from build123d import *

# Parameters (mm, degrees)
SKETCH1_R                  = 35
SKETCH1_R_2                = 13
SKETCH1_R_3                = 5
SKETCH1_R_4                = 2.3
SKETCH1_W                  = 47.96
SKETCH1_H                  = 25
BOSS_EXTRUDE3_DEPTH        = 5.588
F_4_6_4_6_DIAMETER_HOLE1_D = 4.6
FILLET1_R                  = 3
FILLET2_R                  = 2
FILLET3_R                  = 2
FILLET4_R                  = 1
SKETCH6_W                  = 55.082421743
SKETCH6_H                  = 3.3
CUT_EXTRUDE5_DEPTH         = 10
SKETCH7_W                  = 1.65
SKETCH7_H                  = 1.65
BOSS_EXTRUDE4_DEPTH        = 5.588
FILLET5_R                  = 1
FILLET6_R                  = 0.5
FILLET7_R                  = 0.5
FILLET11_R                 = 1
FILLET13_R                 = 0.1
FILLET14_R                 = 0.1


with BuildPart() as part:
    # Sketch1 → Boss-Extrude3 (new body)
    # profile 1 of 5: a face of its own
    with BuildSketch(Plane(origin=(0, 0, 0), x_dir=(1, 0, 0), z_dir=(0, 1, 0))):
        with Locations((32.785, 23.351471482)):
            Circle(SKETCH1_R)
        with Locations(Location((32.785, 23.351471482, 0), (0, 0, 270))):
            Circle(SKETCH1_R_2, mode=Mode.SUBTRACT)
    # profile 2 of 5: a face of its own
    with BuildSketch(Plane(origin=(0, 0, 0), x_dir=(1, 0, 0), z_dir=(0, 1, 0))):
        with Locations((65.600049901, 5.201471482)):
            Circle(SKETCH1_R_3)
        with Locations(Location((65.600049901, 5.201471482, 0), (0, 0, 270))):
            Circle(SKETCH1_R_4, mode=Mode.SUBTRACT)
    # profile 3 of 5: a face of its own
    with BuildSketch(Plane(origin=(0, 0, 0), x_dir=(1, 0, 0), z_dir=(0, 1, 0))):
        with Locations((-0.030049901, 5.201471482)):
            Circle(SKETCH1_R_3)
        with Locations(Location((-0.030049901, 5.201471482, 0), (0, 0, 270))):
            Circle(SKETCH1_R_4, mode=Mode.SUBTRACT)
    # profile 4 of 5: a face of its own
    with BuildSketch(Plane(origin=(0, 0, 0), x_dir=(1, 0, 0), z_dir=(0, 1, 0))):
        with Locations((32.785, 68.701471482)):
            Circle(SKETCH1_R_3)
    # profile 5 of 5: a face of its own
    with BuildSketch(Plane(origin=(0, 0, 0), x_dir=(1, 0, 0), z_dir=(0, 1, 0))):
        with Locations((32.785, 54.201471482)):
            Rectangle(SKETCH1_W, SKETCH1_H)
    extrude(amount=BOSS_EXTRUDE3_DEPTH)

    # Ø4.6 (4.6) Diameter Hole1 (through all)
    with Locations(Plane(origin=(0, 5.588, 0), x_dir=(1, 0, 0), z_dir=(0, 1, 0))):
        with Locations((32.785, 68.701471482)):
            Hole(F_4_6_4_6_DIAMETER_HOLE1_D / 2)

    # Fillet1
    fillet1_edges = [part.edges().sort_by_distance(p)[0] for p in [
        (65.214711372, 2.794, -10.18660079),
        (61.172514444, 2.794, -2.878342174),
        (0.355288628, 2.794, -10.18660079),
        (4.397485556, 2.794, -2.878342174),
    ]]
    fillet(fillet1_edges, radius=FILLET1_R)

    # Fillet2
    fillet2_edges = [part.edges().sort_by_distance(p)[0] for p in [
        (28.202424305, 2.794, -66.701471482),
        (37.367575695, 2.794, -66.701471482),
    ]]
    fillet(fillet2_edges, radius=FILLET2_R)

    # Fillet3
    fillet3_edges = [part.edges().sort_by_distance(p)[0] for p in [
        (8.805, 2.794, -48.845776728),
        (56.765, 2.794, -48.845776728),
    ]]
    fillet(fillet3_edges, radius=FILLET3_R)

    # Fillet4
    fillet4_edges = [part.edges().sort_by_distance(p)[0] for p in [
        (56.765, 2.794, -66.701471482),
        (8.805, 2.794, -66.701471482),
    ]]
    fillet(fillet4_edges, radius=FILLET4_R)

    # Sketch6 → Cut-Extrude5 (cut)
    with BuildSketch(Plane(origin=(0, 5.588, 0), x_dir=(1, 0, 0), z_dir=(0, 1, 0))):
        with Locations((41.000226715, 37.751471482)):
            Rectangle(SKETCH6_W, SKETCH6_H)
    extrude(amount=-CUT_EXTRUDE5_DEPTH, mode=Mode.SUBTRACT)

    # Sketch7 → Boss-Extrude4 (add)
    with BuildSketch(Plane(origin=(0, 5.588, 0), x_dir=(1, 0, 0), z_dir=(0, 1, 0))):
        with Locations((40.61, 38.576471482)):
            Rectangle(SKETCH7_W, SKETCH7_H)
        with Locations((25.56, 38.576471482)):
            Rectangle(SKETCH7_W, SKETCH7_H)
    extrude(amount=-BOSS_EXTRUDE4_DEPTH)

    # Fillet5
    fillet5_edges = [part.edges().sort_by_distance(p)[0] for p in [
        (13.459015843, 2.794, -36.101471482),
        (13.459015843, 2.794, -39.401471482),
    ]]
    fillet(fillet5_edges, radius=FILLET5_R)

    # Fillet6
    fillet6_edges = [part.edges().sort_by_distance(p)[0] for p in [
        (26.385, 2.794, -39.401471482),
        (24.735, 2.794, -39.401471482),
        (41.435, 2.794, -39.401471482),
        (39.785, 2.794, -39.401471482),
    ]]
    fillet(fillet6_edges, radius=FILLET6_R)

    # Fillet7
    fillet7_edges = [part.edges().sort_by_distance(p)[0] for p in [
        (26.385, 2.794, -37.751471482),
        (24.735, 2.794, -37.751471482),
        (41.435, 2.794, -37.751471482),
        (39.785, 2.794, -37.751471482),
    ]]
    fillet(fillet7_edges, radius=FILLET7_R)

    # Fillet11
    fillet11_edges = [part.edges().sort_by_distance(p)[0] for p in [
        (63.888014323, 2.794, -39.401471482),
        (65.380053306, 2.794, -36.101471482),
    ]]
    fillet(fillet11_edges, radius=FILLET11_R)

    # Fillet13
    fillet13_edges = [part.edges().sort_by_distance(p)[0] for p in [
        (30.247777109, 2.794, -36.101471482),
    ]]
    fillet(fillet13_edges, radius=FILLET13_R)

    # Fillet14
    fillet14_edges = [part.edges().sort_by_distance(p)[0] for p in [
        (35.322222891, 2.794, -36.101471482),
    ]]
    fillet(fillet14_edges, radius=FILLET14_R)


solid = part.part
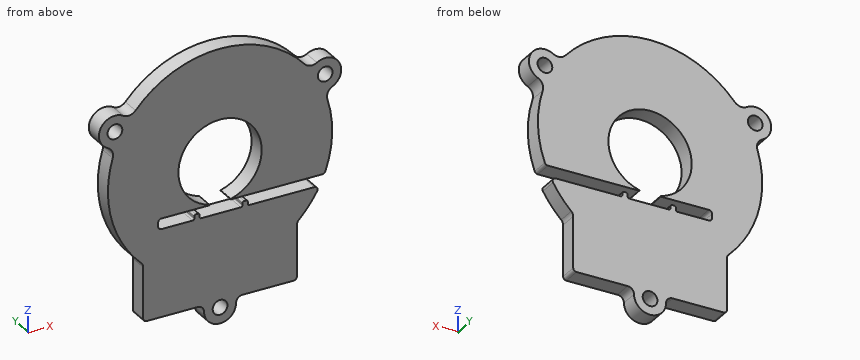
Can you work these out from the model? Positions are in its coordinate system, mm. Give positions to 0.01 mm unless a question says otherwise; leave off trailing zeros. Order: outer loops, then holes, each group sorted by start corner. A loop starts at its lowest first (then second) coordinate and runs counter-clockwise, first axis right, second up. Notation, with made-up numbers: M -10,0 L 47,0 A22 cw 47,10 Z; hole C -14,-40 d2. An arc over 180 degrees is marked long. Use a Markdown table: item, result. Add a question column.
Item 1: If I drill on L1, parallel to Z at x = 44, y = 1.2; L2, parallel to Z at x = 32, y = 1.8; L3, parallel to X at y = 2.5, z = -51.5 (3 decimals), over which ranges is the centre line in solid material (lowest first)? Write a range as [from, to].
Item 2: Suppose I cut it at B-B (z = -4). List the corners of the cut face in (x, y) for me.
Item 3: Suppose I cut it at D-D (z = -58). List the corners of the cut face in (x, y) for me (3 decimals), then the cut area to 3 significant figures.
Item 4: Suppose I cut it at A-A (x = 51). List the corners of the cut face in (y, z) for me, then the cut area to 3 significant figures.
Item 5: Suppose I cut it at C-C (x = 43). List the corners of the cut face in (y, z) for me, then the cut area to 3 significant figures.
Item 6: Will these pins go through, and if not, where does the flat tip stop? pin 1 (3 mm diameter, centred on x = 50.5, y = 3, fed in from -Z); pin 2 (4 mm diameter, centred on x = -0.03, z = -5.2, fed in from -Y); pin 3 (0.7 mm diameter, centred on y = 2, z = -38.5, fed in from +X) (3 decimals); pin 4 (7.5 mm diameter, centred on x = 32.78, z = -68.7, fed in from -Y).
Answer sheet:
| question | item | result |
|---|---|---|
| 1 | L1 | z = [-66.7, -39.4], [-36.1, -29.93], [-16.78, 9.8] |
| 1 | L2 | z = [-73.64, -70.86], [-66.54, -39.4], [-10.38, 11.64] |
| 1 | L3 | x = [8.805, 56.765] |
| 2 | outline | M -4.88,0 L -1.99,0 L -1.99,5.59 L -4.88,5.59 Z; M 1.93,0 L 63.64,0 L 63.64,5.59 L 1.93,5.59 Z; M 67.56,0 L 70.45,0 L 70.45,5.59 L 67.56,5.59 Z |
| 3 | outline | M 8.805,0 L 56.765,0 L 56.765,5.588 L 8.805,5.588 Z |
| 3 | area | 268 mm² |
| 4 | outline | M 0,-66.7 L 5.59,-66.7 L 5.59,-39.4 L 0,-39.4 Z; M 0,-36.1 L 5.59,-36.1 L 5.59,6.54 L 0,6.54 Z |
| 4 | area | 391 mm² |
| 5 | outline | M 0,-66.7 L 5.59,-66.7 L 5.59,-39.4 L 0,-39.4 Z; M 0,-36.1 L 5.59,-36.1 L 5.59,-31.39 L 0,-31.39 Z; M 0,-15.31 L 5.59,-15.31 L 5.59,10.12 L 0,10.12 Z |
| 5 | area | 321 mm² |
| 6 | pin 1 | stops at z = -66.7 |
| 6 | pin 2 | passes through |
| 6 | pin 3 | stops at x = 41.435 |
| 6 | pin 4 | stops at y = 0 |
